The figure shows three views and two pictorial views of one solid part (mm, origin at its lowest corner). Answer the questions. Coordinates: 2 decimals unless noted, no trailing zeros. Use one line per item in the form item = value.
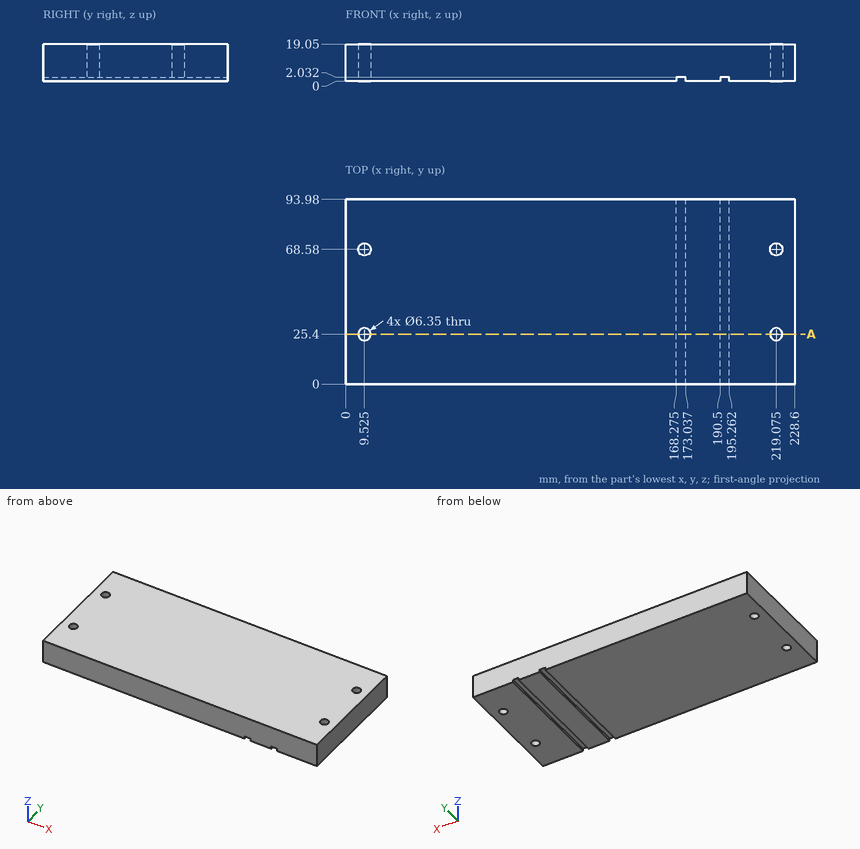
(1) Each of these flat-tipped pins is pushed along its axis until it touches: P1, Ø2.5, axis at x = 193.5, y = 34.5, coming from the -Z side; P2, Ø5, axis at x = 219.075, y = 25.4, coming from the -Z side; P3, Ø2, axis at x = 136, z = 15.5, coming from the -Y side. Where does it stop, or does it pass through?
Data:
P1 = 2.03
P2 = through
P3 = 0
(2) Section A-A on y = 25.4 is taken. Count the separate pieces of the cut face and the enclosed holes in it, plus the area to 3 significant figures.
Data:
separate_pieces = 3
enclosed_holes = 0
area = 4,090 mm²
(3) Straight lines are drawn through the part: line 1 along X through (y, z) = (68.58, 10.5); line 2 along Z through (x, y) = (169, 29). For each, find the intervals that lie inside material, in ascending order.
Data:
line_1 = 0 to 6.35, 12.7 to 215.9, 222.25 to 228.6
line_2 = 2.03 to 19.05
